from build123d import *

# Parameters (mm, degrees)
F1_DEPTH  = 11.176
F2_W      = 15.24
F2_H      = 14.224
F3_DEPTH  = 14.224
F4_R      = 2.413
F5_DEPTH  = 14.225
F7_DEPTH  = 14.225
F9_DEPTH  = 14.225
F10_W     = 69.088
F10_H     = 23.9414346935
F11_DEPTH = 11.177


with BuildPart() as f1:
    # F0 (on Top) → F1 (new body)
    with BuildSketch(Plane.XY):
        with BuildLine():
            Line((36.576, -66.802), (41.148, -66.802))
            Line((41.148, -66.802), (41.148, -18.9191306131))
            ThreePointArc((41.148, -18.9191306131), (43.9343121331, -7.9817335086), (51.6140240964, 0.2894341771))
            ThreePointArc((51.6140240964, 0.2894341771), (60.2346282504, 19.3987779476), (46.3452307692, 35.1012132022))
            ThreePointArc((46.3452307692, 35.1012132022), (42.5943851715, 37.6516131673), (41.148, 41.9506075399))
            Line((41.148, 41.9506075399), (41.148, 66.802))
            Line((41.148, 66.802), (36.576, 66.802))
            Line((36.576, 66.802), (-36.576, 66.802))
            Line((-36.576, 66.802), (-41.148, 66.802))
            Line((-41.148, 66.802), (-41.148, 41.5621785081))
            ThreePointArc((-41.148, 41.5621785081), (-42.5208525009, 37.5313086462), (-46.068627451, 35.1763290844))
            ThreePointArc((-46.068627451, 35.1763290844), (-60.2126563181, 19.5403952666), (-51.6140240964, 0.2894341771))
            ThreePointArc((-51.6140240964, 0.2894341771), (-43.9343121331, -7.9817335086), (-41.148, -18.9191306131))
            Line((-41.148, -18.9191306131), (-41.148, -66.802))
            Line((-41.148, -66.802), (-36.576, -66.802))
            Line((-36.576, -66.802), (36.576, -66.802))
        make_face()
        with BuildLine():
            ThreePointArc((-41.148, 11.684), (-45.974, 16.51), (-41.148, 21.336))
            Line((-41.148, 21.336), (41.148, 21.336))
            ThreePointArc((41.148, 21.336), (45.974, 16.51), (41.148, 11.684))
            Line((41.148, 11.684), (-41.148, 11.684))
        make_face(mode=Mode.SUBTRACT)
    extrude(amount=F1_DEPTH)

    # F2 (on face) → F3 (join)
    with BuildSketch(Plane.XY.offset(11.176)):
        with Locations((-33.528, 59.69)):
            Rectangle(F2_W, F2_H)
        with Locations((33.528, 59.69)):
            Rectangle(F2_W, F2_H)
    extrude(amount=F3_DEPTH)

    # F4 (on face) → F5 (cut, through all)
    with BuildSketch(Plane.XZ.offset(-52.578)):
        with Locations((-33.528, 17.78)):
            Circle(F4_R)
        with Locations((33.528, 17.78)):
            Circle(F4_R)
    extrude(amount=-F5_DEPTH, mode=Mode.SUBTRACT)

    # F6 (on face) → F7 (cut, through all)
    with BuildSketch(Plane.XZ.offset(-52.578)):
        with BuildLine():
            ThreePointArc((33.528, 25.4), (38.9161536726, 23.1681536726), (41.148, 17.78))
            Line((41.148, 17.78), (41.148, 25.4))
            Line((41.148, 25.4), (33.528, 25.4))
        make_face()
        with BuildLine():
            ThreePointArc((25.908, 17.78), (28.1398463274, 23.1681536726), (33.528, 25.4))
            Line((33.528, 25.4), (25.908, 25.4))
            Line((25.908, 25.4), (25.908, 17.78))
        make_face()
    extrude(amount=-F7_DEPTH, mode=Mode.SUBTRACT)

    # F8 (on face) → F9 (cut, through all)
    with BuildSketch(Plane.XZ.offset(-52.578)):
        with BuildLine():
            ThreePointArc((-41.148, 17.78), (-38.9161536726, 23.1681536726), (-33.528, 25.4))
            Line((-33.528, 25.4), (-41.148, 25.4))
            Line((-41.148, 25.4), (-41.148, 17.78))
        make_face()
        with BuildLine():
            ThreePointArc((-33.528, 25.4), (-28.1398463274, 23.1681536726), (-25.908, 17.78))
            Line((-25.908, 17.78), (-25.908, 25.4))
            Line((-25.908, 25.4), (-33.528, 25.4))
        make_face()
    extrude(amount=-F9_DEPTH, mode=Mode.SUBTRACT)

    # F10 (on face) → F11 (cut, through all)
    with BuildSketch(Plane.XY.offset(11.176)):
        with Locations((0, -54.8312826533)):
            Rectangle(F10_W, F10_H)
    extrude(amount=-F11_DEPTH, mode=Mode.SUBTRACT)


solid = f1.part
Input: part model. Units: mm. Frame: model coordinates. A direction names the side the tool comes from. Give positions to 0.01 mm unless a question says otherwise; leave off trailing zeros. Order: outer loops, then holes, each group sorted by start corner. A loop starts at its lowest first (then second) coordinate and runs counter-clockwise, first axis right, second up. Notation, with made-up numbers: (-16, 30) - (25, 30) arc R12 ccw to (25, 43) - close; hole circle Ø1 at (40.25, 18). An arc over 180 degrees is marked (long way). Write each question's results on one line, items separated by ' | '.
Item 1: Material intervals for line 1 along Z through (x, y) = (3, 51.5); line 2 along Y through (x, z) = (-20.5, 2); line 3 along Y through (x, z) = (37, 6), sorted ascending.
A:
line 1: z = 0 to 11.18 | line 2: y = -42.86 to 11.68, 21.34 to 66.8 | line 3: y = -66.8 to 11.68, 21.34 to 66.8
Item 2: Section D-D (y = -36). Return loops of the section in (x, z).
A:
outline: (-41.15, 0) - (41.15, 0) - (41.15, 11.18) - (-41.15, 11.18) - close
Item 3: Section A-A (y = 16.51). Return loops of the section in (x, z), and give its area (3 significant figures).
A:
outline: (-60.45, 0) - (-45.97, 0) - (-45.97, 11.18) - (-60.45, 11.18) - close; (45.97, 0) - (60.45, 0) - (60.45, 11.18) - (45.97, 11.18) - close | area: 324 mm^2
Item 4: Draft query along X for faces 4 (the cylindrical face through (-60.16, 19.85, 5.51)), 5 (the flat face through (41.148, -43, 6)), 6 (the cylindrical face through (45.973, 16.616, 5.51)), 7 (the flat face through (38, -66.802, 6)). Return one class per face: released by +X, released by -X, zero draft, split by the parting line, or undercut.
A:
face 4: released by -X | face 5: released by +X | face 6: undercut | face 7: zero draft
Item 5: Contact query for flat-ended pins moving along their axis: pin 1 Ø7.5 at (y, z) = (56, 14) entering from -X; pin 2 Ø3 at (x, y) = (7, -32) entering from +Z; pin 3 Ø4.5 at (x, z) = (32.5, 20) entering from -Y. Output: stop coordinate, or through.
A:
pin 1: stops at x = -41.15 | pin 2: stops at z = 11.18 | pin 3: stops at y = 52.58
Item 6: Section C-C (z = 5). Return loops of the section in (x, y), and give its area (3 significant figures).
A:
outline: (-51.61, 0.29) arc R22.86 cw to (-41.15, -18.92) - (-41.15, -66.8) - (-34.54, -66.8) - (-34.54, -42.86) - (34.54, -42.86) - (34.54, -66.8) - (41.15, -66.8) - (41.15, -18.92) arc R22.86 cw to (51.61, 0.29) arc R19.3 ccw to (46.35, 35.1) arc R7.11 cw to (41.15, 41.95) - (41.15, 66.8) - (-41.15, 66.8) - (-41.15, 41.56) arc R6.6 cw to (-46.07, 35.18) arc R19.3 ccw to start; hole (-41.15, 11.68) - (41.15, 11.68) arc R4.83 ccw to (41.15, 21.34) - (-41.15, 21.34) arc R4.83 ccw to start | area: 9,730 mm^2
Item 7: Access query for faces 1 (the flat face through (-32, 52.578, 20)), 2 (the flat face through (25.908, 60, 14)), 3 (the flat face through (1, 11.684, 6)). Directions: +Z, -Z, +X, -X, +Y, -Y. A direction counts if a zero-diameter tool reaches every point of the face in a straight line with its end or side. Return the directions, or none.
A:
face 1: +Z, +X, -X, -Y | face 2: +Z, +Y, -Y | face 3: +Z, -Z
Item 8: Section B-B (x = -13). Return loops of the section in (y, z), and give its area (3 significant figures).
A:
outline: (-42.86, 0) - (11.68, 0) - (11.68, 11.18) - (-42.86, 11.18) - close; (21.34, 0) - (66.8, 0) - (66.8, 11.18) - (21.34, 11.18) - close | area: 1,120 mm^2
